Autodesk Inventor part; units mm, degrees
ref_plane "YZ Plane" through (0, 0, 0) normal (1, 0, 0) x (0, 1, 0)
ref_plane "XZ Plane" through (0, 0, 0) normal (0, 1, 0) x (-1, 0, 0)
ref_plane "XY Plane" through (0, 0, 0) normal (0, 0, 1) x (1, 0, 0)
sketch "Sketch1" plane through (0, 0, 0) normal (1, 0, 0) x (0, 1, 0)
  line L0 (0, 0) -> (44.45, 0)
  line L1 (44.45, 0) -> (44.45, -19.05)
  line L2 (44.45, -19.05) -> (0, -19.05)
  line L3 (0, -19.05) -> (0, 0)
  dimension "d0" = 44.45
  dimension "d1" = 19.05
extrude "Extrusion1" add sketch "Sketch1" along normal blind 44.45
sketch "Sketch2" plane through (0, 0, 0) normal (0, 0, 1) x (1, 0, 0)
  line L0 (0, 0) -> (0, 44.45)
  line L1 (0, 0) -> (44.45, 0)
  line L2 (44.45, 44.45) -> (44.45, 0)
  line L3 (0, 44.45) -> (44.45, 44.45)
  point P0 (22.225, 22.225)
  dimension "d4" = 22.225
  dimension "d5" = 22.225
hole "Hole1" at (22.225, 22.225, 0) direction (0, 0, -1) diameter 6.35 end through all
properties part number "tension_block"
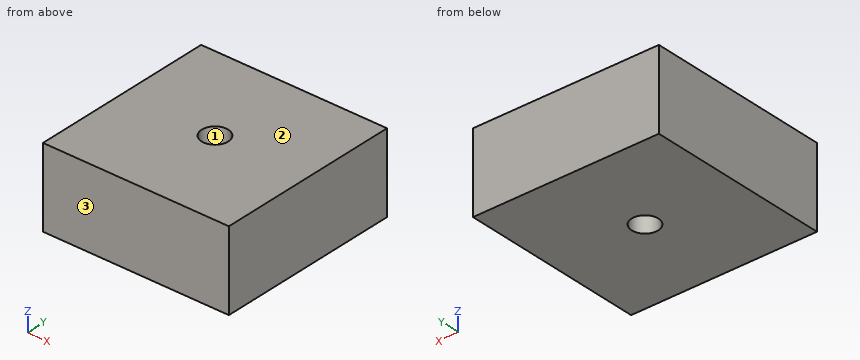
Check sheet for the modelled part. Datum: model origin and axes. Units: mm. Face numbers are marked on the shaded views. Give positions to 0.01 mm unless a question says otherwise; leave off trailing zeros. Order: outer loops, then holes, each group sorted by start corner. A loop starts at its lowest first (then second) coordinate and runs counter-clockwise, first axis right, second up. Notation, with made-up numbers: M -7.75,34.5 L 40.25,34.5 A29 ccw 40.25,58.5 Z; hole C 62.5,85 d4. An arc over 180 degrees is marked long. Answer as CSV lines item,"result". Start each with the question number.
Item 1: Cross-section at B-B on y = 21. Enter the section's corners in (x, z), plus the area to 3 significant figures.
Item 2: Cross-section at C-C on z = -17.25. Enter the section's corners in (x, y) (3 decimals), plus the area to 3 significant figures.
Item 3: Cross-section at A-A on x = 23. Enter the section's corners in (y, z).
Item 4: Thickness scan on line 1 (Y direction, x = 22, z = -13.75); line 2 (X direction, y = 23.5, z = -10.5); line 3 (X direction, y = 21, z = -13.5). Record the ranges inside material, lowest first. Write a range as [from, to].
Item 5: Mould release check, pull along Y, two halves, no side actions. Record for the marked faces 1, 2 and 3: +Y half, -Y half, draft (parallel to the pull), parting line (faces both ways), or undercut.
Established:
1,outline,"M 0,-19.05 L 19.3,-19.05 L 19.3,0 L 0,0 Z; M 25.15,-19.05 L 44.45,-19.05 L 44.45,0 L 25.15,0 Z"
1,area,"735 mm^2"
2,outline,"M 0,0 L 44.45,0 L 44.45,44.45 L 0,44.45 Z; hole C 22.225,22.225 d6.35"
2,area,"1,940 mm^2"
3,outline,"M 0,-19.05 L 19.15,-19.05 L 19.15,0 L 0,0 Z; M 25.3,-19.05 L 44.45,-19.05 L 44.45,0 L 25.3,0 Z"
4,line 1,"y = [0, 19.06], [25.39, 44.45]"
4,line 2,"x = [0, 19.32], [25.13, 44.45]"
4,line 3,"x = [0, 19.3], [25.15, 44.45]"
5,face 1,"undercut"
5,face 2,"draft"
5,face 3,"-Y half"
